Autodesk Fusion 360 part; units mm, degrees
sketch "Sketch1" plane through (0, 0, 0) normal (0, 0, 1) x (1, 0, 0)
  line L0 (0, 0) -> (0, 55) construction
  line L1 (0, 12.5) -> (12.5, 12.5) construction
  arc A0 (0, 0) -> (12.5, 12.5) centre (0, 12.5) ccw
  line L2 (0, 55) -> (12.5, 55)
  line L3 (12.5, 55) -> (12.5, 12.5)
  line L4 (0, 55) -> (-12.5, 55)
  line L5 (-12.5, 55) -> (-12.5, 12.5)
  arc A1 (-12.5, 12.5) -> (0, 0) centre (0, 12.5) ccw
  line L6 (14.5, 55) -> (14.5, 12.5) construction
  line L7 (12.5, 55) -> (14.5, 53)
  line L8 (12.5, 55) -> (26.8265, 55) construction
  line L9 (14.5, 53) -> (14.5, 30)
  line L10 (14.5, 30) -> (12.5, 30)
  line L11 (-14.5, 30) -> (-12.5, 30)
  line L12 (-12.5, 55) -> (-26.8265, 55) construction
  line L13 (-14.5, 53) -> (-14.5, 30)
  line L14 (-14.5, 55) -> (-12.5, 55)
  line L15 (12.5, 55) -> (14.5, 55)
  line L16 (-12.5, 55) -> (-14.5, 53)
  dimension "d1" = 55
  dimension "d2" = 25
  dimension "d4" = 12.5
  dimension "d5" = 2
  dimension "d6" = 45
  dimension "d7" = 25
extrude "Extrude1" add sketch "Sketch1" along normal mid plane 27
sketch "Sketch2" plane through (0, 0, 13.5) normal (0, 0, 1) x (1, 0, 0)
  line L0 (12.5, 55) -> (-12.5, 55)
  line L1 (-12.5, 55) -> (-14.5, 53)
  line L2 (-14.5, 53) -> (-14.5, 30)
  line L3 (-14.5, 30) -> (-12.5, 30)
  line L4 (-12.5, 30) -> (-12.5, 12.5)
  arc A0 (-12.5, 12.5) -> (12.5, 12.5) centre (0, 12.5) ccw
  line L5 (12.5, 12.5) -> (12.5, 30)
  line L6 (12.5, 30) -> (14.5, 30)
  line L7 (14.5, 30) -> (14.5, 53)
  line L8 (14.5, 53) -> (12.5, 55)
  arc A1 (-12.5, 12.5) -> (12.5, 12.5) centre (0, 12.5) ccw
  circle A2 centre (0, 12.5) radius 6
  dimension "d10" = 12
extrude "Extrude2" cut sketch "Sketch2" against normal through all contours A2
sketch "Sketch3" plane through (0, 0, 0) normal (1, 0, 0) x (0, 0, -1)
  line L0 (13.5, 18.5) -> (13.5, 6.5) construction
  line L1 (-13.5, 6.5) -> (-13.5, 18.5) construction
  line L2 (13.5, 55) -> (-13.5, 55) construction
  line L3 (13.5, 30) -> (13.5, 53) construction
  line L4 (13.5, 53) -> (13.5, 55) construction
  line L5 (-13.5, 55) -> (-13.5, 53) construction
  line L6 (-13.5, 53) -> (-13.5, 30) construction
  line L7 (-13.5, 30) -> (-13.5, 12.5) construction
  line L8 (13.5, 12.5) -> (13.5, 30) construction
  line L9 (13.5, 0) -> (13.5, 12.5) construction
  line L10 (-13.5, 12.5) -> (-13.5, 0) construction
  line L11 (13.5, 12.5) -> (-13.5, 12.5) construction
  line L12 (-13.5, 12.5) -> (-13.5, 0) construction
  line L13 (-13.5, 12.5) -> (13.5, 12.5) construction
  line L14 (13.5, 0) -> (13.5, 12.5) construction
  line L15 (13.5, 0) -> (-13.5, 0) construction
  line L16 (-13.5, 42.5) -> (13.5, 42.5) construction
  line L17 (13.5, 32.5) -> (-13.5, 32.5) construction
  line L18 (13.5, 32.5) -> (13.5, 2)
  line L19 (7.5, 31.5) -> (7.5, 0)
  line L20 (11.5, 0) -> (7.5, 0)
  line L21 (0, 32.5) -> (6.5, 32.5)
  arc A0 (7.5, 31.5) -> (6.5, 32.5) centre (6.5, 31.5) ccw
  line L22 (0, 55) -> (0, 0) construction
  circle A1 centre (0, 42.5) radius 12.5 construction
  line L23 (13.5, 42.5) -> (12.4564, 43.5436)
  line L24 (13.5, 42.5) -> (21.4057, 42.5) construction
  arc A2 (12.4564, 43.5436) -> (0, 55) centre (0, 42.5) ccw
  line L25 (13.5, 42.5) -> (13.5, 32.5)
  arc A3 (0, 55) -> (-12.4564, 43.5436) centre (0, 42.5) ccw
  line L26 (-13.5, 42.5) -> (-12.4564, 43.5436)
  line L27 (-13.5, 42.5) -> (-13.5, 32.5)
  line L28 (-13.5, 32.5) -> (-13.5, 2)
  line L29 (-11.5, 0) -> (-7.5, 0)
  line L30 (-7.5, 31.5) -> (-7.5, 0)
  arc A4 (-6.5, 32.5) -> (-7.5, 31.5) centre (-6.5, 31.5) ccw
  line L31 (0, 32.5) -> (-6.5, 32.5)
  line L32 (7.5, 0) -> (-7.5, 0)
  line L33 (-11.5, 0) -> (-13.5, 0)
  line L34 (-13.5, 2) -> (-13.5, 0)
  line L35 (13.5, 2) -> (13.5, 0)
  line L36 (13.5, 0) -> (11.5, 0)
  line L37 (13.5, 55) -> (13.5, 42.5)
  line L38 (13.5, 55) -> (0, 55)
  line L39 (0, 55) -> (-13.5, 55)
  line L40 (-13.5, 55) -> (-13.5, 42.5)
  circle A5 centre (0, 42.5) radius 6
  dimension "d12" = 30
  dimension "d13" = 20
  dimension "d16" = 1
  dimension "d17" = 25
  dimension "d18" = 135
  dimension "d21" = 12
extrude "Extrude3" cut sketch "Sketch3" along normal through all and the other way through all contours L23 A2 L37 L38 | A3 L26 L39 L40 | L19 L21 A0 L30 A4 L31 L32 | A5
fillet "Fillet1" radius 0.5 12 edges at (12.5, 21.25, -13.5) (0, 0, -13.5) (-12.5, 21.25, -13.5) (12.5, 21.25, -7.5) (0, 0, -7.5) (-12.5, 21.25, -7.5) (-12.5, 21.25, 7.5) (0, 0, 7.5) (12.5, 21.25, 7.5) (-12.5, 21.25, 13.5) (0, 0, 13.5) (12.5, 21.25, 13.5)
equation "d1 = 12.5 mm + 30 mm + 12.5 mm"
equation "d2 = ( 12.5 * 2 ) * 1 mm"
equation "d8 = 6 mm + 15 mm + 6 mm"
equation "d17 = ( 12.5 * 2 ) * 1 mm"
Input: part model. Units: mm. Frame: model coordinates. A direction names the side the tool comes from. Give positions to 0.01 mm unless a question says otherwise; leave off trailing zeros. Order: outer loops, then holes, each group sorted by start corner. A loop starts at its lowest first (then second) coordinate and runs counter-clockwise, first axis right, second up. Notation, with made-up numbers: (83, 69.5) -> (114, 69.5) arc R11 ccw to (114, 81.5) -> close; hole circle Ø7 at (-36, 32). An arc over 180 degrees is marked (long way). Use one line per item in the form item = value.
1) Mould query, pull axis Y, two halves, no side actions, for faces 5 (the flat face through (-14, 30, -11)), 6 (the cylindrical face through (0.203, 36.643, 1.301)), 7 (the flat face through (12.5, 21, 10)). Classes: pulls with the +Y half, pulls with the -Y half, needs draft (parallel to the pull), parting line crosses it, or undercut.
Response values:
face_5 = pulls with the -Y half
face_6 = undercut
face_7 = needs draft
2) Line query: probe 1 along Z at (x, y) = (-3.25, 42.5); probe 2 along Y at (x, z) = (-1.5, 0); probe 3 along Z at (x, y) = (-10.5, 24.5). Output: solid intervals per line, ascending.
Response values:
probe_1 = -13.5 to -6, 6 to 13.5
probe_2 = 32.5 to 36.5, 48.5 to 55
probe_3 = -13.5 to -7.5, 7.5 to 13.5
3) Section D-D, the plane z = 10.25. Return loops of the section in (x, y).
Response values:
outline = (-14.5, 30) -> (-12.5, 30) -> (-12.5, 12.5) arc R12.5 ccw to (12.5, 12.5) -> (12.5, 30) -> (14.5, 30) -> (14.5, 49.65) -> (-14.5, 49.65) -> close; hole circle Ø12 at (0, 12.5)
4) Section A-A, the plane x = 0. Return loops of the section in (y, z).
Response values:
outline = (0, -13) arc R0.5 ccw to (0.5, -13.5) -> (6.5, -13.5) -> (6.5, -7.5) -> (0.5, -7.5) arc R0.5 ccw to (0, -8) -> close; (0, 8) arc R0.5 ccw to (0.5, 7.5) -> (6.5, 7.5) -> (6.5, 13.5) -> (0.5, 13.5) arc R0.5 ccw to (0, 13) -> close; (18.5, -13.5) -> (42.5, -13.5) -> (43.54, -12.46) arc R12.5 ccw to (55, 0) arc R12.5 ccw to (43.54, 12.46) -> (42.5, 13.5) -> (18.5, 13.5) -> (18.5, 7.5) -> (31.5, 7.5) arc R1 cw to (32.5, 6.5) -> (32.5, -6.5) arc R1 cw to (31.5, -7.5) -> (18.5, -7.5) -> close; hole circle Ø12 at (42.5, 0)
5) First-contact query: pin 1 Ø3 at (x, z) = (-12.5, 9) entering from -Y; pin 2 Ø3 at (x, z) = (13, 11.5) entering from -Y; pin 3 Ø1.5 at (y, z) = (25.5, 11) entering from -X. Flat tips, straight axial feed; report the tip coordinate or a pass-through.
Response values:
pin_1 = 6.56
pin_2 = 7.6
pin_3 = -12.5
6) Section B-B, the plane y = 27.5. Return loops of the section in (x, z).
Response values:
outline = (-12.5, -13) arc R0.5 ccw to (-12, -13.5) -> (12, -13.5) arc R0.5 ccw to (12.5, -13) -> (12.5, -8) arc R0.5 ccw to (12, -7.5) -> (-12, -7.5) arc R0.5 ccw to (-12.5, -8) -> close; (-12.5, 8) arc R0.5 ccw to (-12, 7.5) -> (12, 7.5) arc R0.5 ccw to (12.5, 8) -> (12.5, 13) arc R0.5 ccw to (12, 13.5) -> (-12, 13.5) arc R0.5 ccw to (-12.5, 13) -> close
7) Section C-C, the plane z = -1.5. Return loops of the section in (x, y).
Response values:
outline = (-14.5, 32.5) -> (14.5, 32.5) -> (14.5, 36.69) -> (-14.5, 36.69) -> close; (-14.5, 48.31) -> (14.5, 48.31) -> (14.5, 53) -> (12.59, 54.91) -> (-12.59, 54.91) -> (-14.5, 53) -> close
8) Reachability of faces 1 (the flat face through (0, 20, -7.5)), 2 (the flat face through (0, 43, -13)), 3 (the flat face through (12.5, 21, -11)), 4 (the flat face through (-12.5, 21, 10)) from +Z, -Z, +X, -X, +Y, -Y: full face, straight path, thin tool, end or side. Return the list, or none.
Response values:
face_1 = +X, -X, -Y
face_2 = -Z, +X, -X, +Y
face_3 = +Z, -Z, +X, -Y
face_4 = +Z, -Z, -X, -Y
